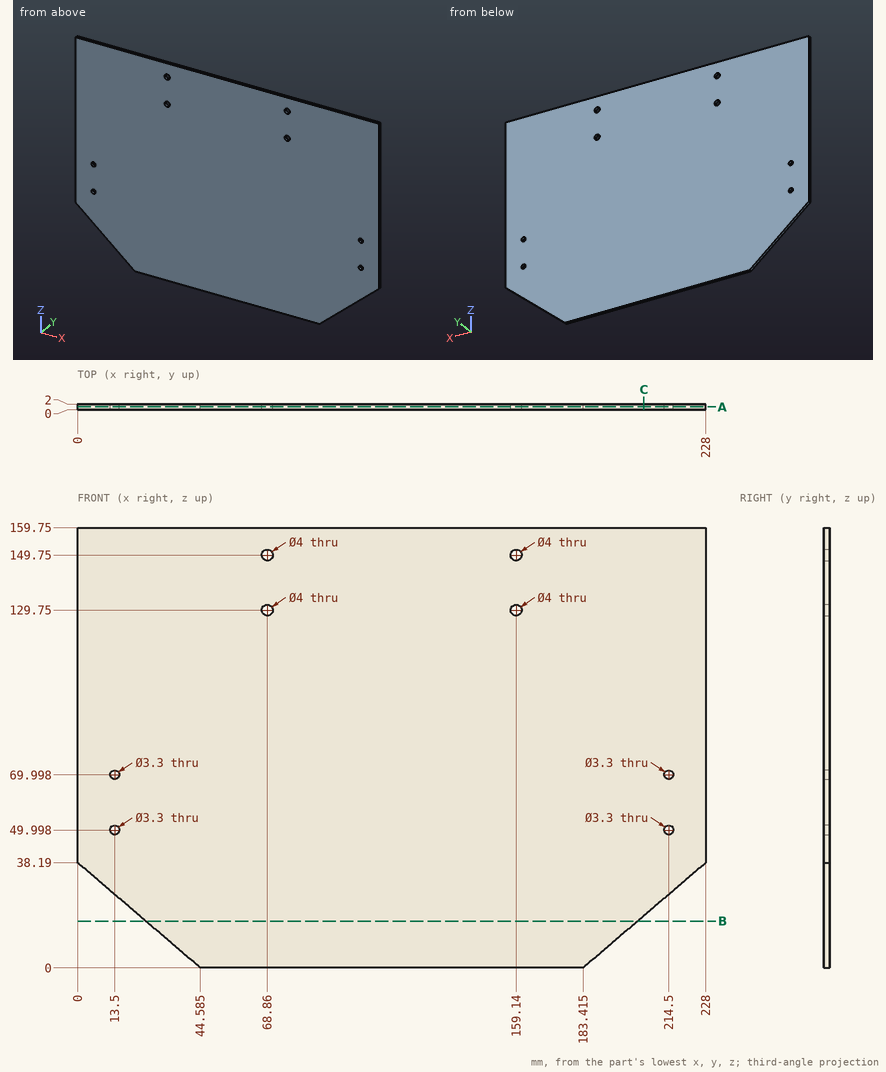
Print and shaded views of the part. All mm, measured from the part's lowest x, y and z. Round coordinates to 2 decimals unless told otherwise and drop trailing zeros. Loops run counter-clockwise (first coordinate to the right, second up) from the corner with the lowest first, then second, coordinate; pieces in that order, holes last. Notation, with made-up numbers: M -33.75,49 L -7.75,49 A30 cw -7.75,84 Z; hole C 45.25,49 d11. An arc over 180 degrees is marked long. One line per question, with ' | ' between items.
1) Drill centre lines: line 1 along Z through (x, y) = (159.14, 0.65); line 2 along X through (y, z) = (0.85, 129.75); line 3 along X through (y, z) = (0.4, 128). Where is each one in solid material? Low to high.
Solved:
line 1: z = 0 to 127.75, 131.75 to 147.75, 151.75 to 159.75 | line 2: x = 0 to 66.86, 70.86 to 157.14, 161.14 to 228 | line 3: x = 0 to 67.89, 69.83 to 158.17, 160.11 to 228
2) Band-saw the part on B-B (z = 17). Give the cut face in (x, y).
Solved:
outline: M 24.74,0 L 203.26,0 L 203.26,2 L 24.74,2 Z
3) Band-saw the part on C-C (x = 205.5). Give the cut face in (y, z), then the cut area to 3 significant figures.
Solved:
outline: M 0,18.92 L 2,18.92 L 2,159.75 L 0,159.75 Z | area: 282 mm²
4) Band-saw the part on A-A (y = 0.95). Give the number of separate pieces and of enclosed holes in the cut face, then the cut area to 3 significant figures.
Solved:
separate pieces: 1 | enclosed holes: 8 | area: 34,600 mm²
